from build123d import *

# Parameters (mm, degrees)
ESQUISSE1_W                   = 155
ESQUISSE1_H                   = 155
BOSS_EXTRU_1_DEPTH            = 6.35
ESQUISSE3_R                   = 3.4417
LAZY_SUSAN_BOLT_PATTERN_DEPTH = 6.35
ESQUISSE4_R                   = 7.9375
ENL_V_MAT_EXTRU_2_DEPTH       = 6.35
D_GAGEMENT_M41_D              = 4.8
D_GAGEMENT_M31_D              = 3.6


with BuildPart() as part:
    # Esquisse1 → Boss.-Extru.1 (new body)
    with BuildSketch(Plane(origin=(0, 0, 0), x_dir=(1, 0, 0), z_dir=(0, 1, 0))):
        Rectangle(ESQUISSE1_W, ESQUISSE1_H)
    extrude(amount=BOSS_EXTRU_1_DEPTH)

    # Esquisse3 → lazy_susan_bolt_pattern (cut)
    with BuildSketch(Plane(origin=(0, 6.35, 0), x_dir=(1, 0, 0), z_dir=(0, 1, 0))):
        with Locations(Location((-70.65, 70.65, 0), (0, 0, 270))):
            Circle(ESQUISSE3_R)
        with Locations(Location((70.65, 70.65, 0), (0, 0, 270))):
            Circle(ESQUISSE3_R)
        with Locations(Location((70.65, -70.65, 0), (0, 0, 270))):
            Circle(ESQUISSE3_R)
        with Locations(Location((-70.65, -70.65, 0), (0, 0, 270))):
            Circle(ESQUISSE3_R)
    extrude(amount=-LAZY_SUSAN_BOLT_PATTERN_DEPTH, mode=Mode.SUBTRACT)

    # Esquisse4 → Enlèv. mat.-Extru.2 (cut)
    with BuildSketch(Plane(origin=(0, 6.35, 0), x_dir=(1, 0, 0), z_dir=(0, 1, 0))):
        with Locations(Location((0, 0, 0), (0, 0, 270))):
            Circle(ESQUISSE4_R)
    extrude(amount=-ENL_V_MAT_EXTRU_2_DEPTH, mode=Mode.SUBTRACT)

    # Dégagement M41 (through all)
    with Locations(Plane(origin=(0, 6.35, 0), x_dir=(1, 0, 0), z_dir=(0, 1, 0))):
        with Locations((-34, 34), (34, 34), (34, -34), (-34, -34)):
            Hole(D_GAGEMENT_M41_D / 2)

    # Dégagement M31 (through all)
    with Locations(Plane(origin=(0, 6.35, 0), x_dir=(1, 0, 0), z_dir=(0, 1, 0))):
        with Locations((16.215, 0), (-16.215, 0)):
            Hole(D_GAGEMENT_M31_D / 2)


solid = part.part
For this review, take the finished solid that the model builds, in its own axes (mm). Give positions to 0.01 mm unless a question says otherwise; leave off trailing zeros. Loops run counter-clockwise (first coordinate to the right, second up) from the corner with the lowest first, then second, coordinate; pieces in that order, holes last. Notation, with made-up numbers: M 8.25,-1 L 64.25,-1 A31 ccw 64.25,32 Z; hole C 86.5,83.25 d4. An arc over 180 degrees is marked long. Put each result on its own line as item: value. Start each with the question number.
(1) Add section C-C, the plane x = 0. Write out the cut boundary in (y, z).
(2) Add section A-A, the plane x = -70.65. Write out the cut boundary in (y, z).
(3) Wall thickness on L1, parallel to Z at x = 34, y = 4: over which ranges is the line inside the solid? List them lowest first.
(4) For pin 1 (9 mm diameter, centred on x = -70.65, z = -70.65, fed in from -Y), flat-tipped, find the tip position at first contact; note if it passes through.
(5) The part is to be moulded in two halves that separate along X. For faces 1 (the flat face through (-1, 0, 16)), 2 (the flat face through (-77.5, 3, 1)), 3 (the cylindrical face through (-7.75, 3.22, -1.72)), say which applies: +X half, -X half, draft (parallel to the pull), parting line (faces both ways), or undercut.
(6) Add section B-B, the plane z = 0. Give the number of separate pieces and of enclosed holes in the cut face, then the cut area to 3 significant figures.
(7) Add section D-D, the plane z = -70.65. Write out the cut boundary in (x, y).
Result:
1. outline: M 0,-77.5 L 6.35,-77.5 L 6.35,-7.94 L 0,-7.94 Z; M 0,7.94 L 6.35,7.94 L 6.35,77.5 L 0,77.5 Z
2. outline: M 0,-77.5 L 6.35,-77.5 L 6.35,-74.09 L 0,-74.09 Z; M 0,-67.21 L 6.35,-67.21 L 6.35,67.21 L 0,67.21 Z; M 0,74.09 L 6.35,74.09 L 6.35,77.5 L 0,77.5 Z
3. L1: z = -77.5 to -36.4, -31.6 to 31.6, 36.4 to 77.5
4. pin 1: stops at y = 0
5. face 1: draft
5. face 2: -X half
5. face 3: undercut
6. separate pieces: 4
6. enclosed holes: 0
6. area: 838 mm^2
7. outline: M -77.5,0 L -74.09,0 L -74.09,6.35 L -77.5,6.35 Z; M -67.21,0 L 67.21,0 L 67.21,6.35 L -67.21,6.35 Z; M 74.09,0 L 77.5,0 L 77.5,6.35 L 74.09,6.35 Z
